Design review of the part built by this model. Coordinates are the model's own, in mm. Face numbers are marked on the shaded views. A direction names the side the tool comes from. Coordinates: 2 decimals unless noted, no trailing zeros. Order: outer loops, then holes, each group sorted by start corner. A loop starts at its lowest first (then second) coordinate and runs counter-clockwise, first axis right, second up. Notation, with made-up numbers: (9, 22.25) -> (35, 22.25) arc R31 ccw to (35, 48.25) -> close; hole circle Ø8 at (9, 8). An arc over 180 degrees is marked (long way). Write item = value, one per line.
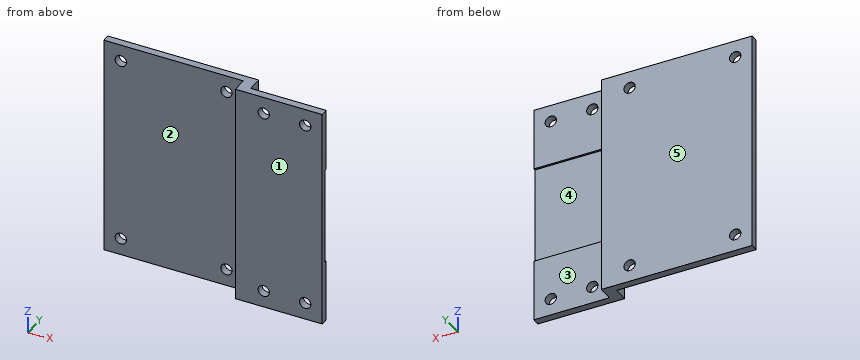
```python
from build123d import *

# Parameters (mm, degrees)
SKETCH_1_W          = 62
SKETCH_1_H          = 59
EXTRUDE_1_DEPTH     = 2
SKETCH_2_W          = 3
SKETCH_2_H          = 59
EXTRUDE_2_DEPTH     = 4
SKETCH_3_W          = 59
SKETCH_3_H          = 2
EXTRUDE_3_DEPTH     = 20
HOLE_WIZARD_M3_2_D  = 3
HOLE_WIZARD_M3_1_D  = 3
SKETCH_6_R          = 1.5
CUT_EXTRUDE_3_DEPTH = 10
SKETCH_7_W          = 59
SKETCH_7_H          = 2
CUT_EXTRUDE_4_DEPTH = 22
HOLE_WIZARD_M3_3_D  = 3
CUT_EXTRUDE_6_DEPTH = 0.5


with BuildPart() as part:
    # Sketch 1 → Extrude 1 (new body)
    with BuildSketch(Plane(origin=(0, 0, 0), x_dir=(1, 0, 0), z_dir=(0, 1, 0))):
        Rectangle(SKETCH_1_W, SKETCH_1_H)
    extrude(amount=EXTRUDE_1_DEPTH)

    # Sketch 2 → Extrude 2 (add)
    with BuildSketch(Plane.XZ):
        with Locations((29.5, 0)):
            Rectangle(SKETCH_2_W, SKETCH_2_H)
    extrude(amount=EXTRUDE_2_DEPTH)

    # Sketch 3 → Extrude 3 (add)
    with BuildSketch(Plane(origin=(31, 0, 0), x_dir=(0, 0, -1), z_dir=(1, 0, 0))):
        with Locations((0, -3)):
            Rectangle(SKETCH_3_W, SKETCH_3_H)
    extrude(amount=EXTRUDE_3_DEPTH)

    # Hole Wizard M3 _2 (through all)
    with Locations(Plane(origin=(23.5, 2, -25), x_dir=(0, 0, 1), z_dir=(0, 1, 0))):
        with Locations((0, 0), (50, 0)):
            Hole(HOLE_WIZARD_M3_2_D / 2)

    # Hole Wizard M3 _1 (through all)
    with Locations(Plane(origin=(35.5, -2, -25), x_dir=(0, 0, 1), z_dir=(0, 1, 0))):
        with Locations((0, 0), (0, 11), (50, 0), (50, 11)):
            Hole(HOLE_WIZARD_M3_1_D / 2)

    # Sketch 6 → Cut-Extrude 3 (cut)
    with BuildSketch(Plane(origin=(0, 2, 0), x_dir=(1, 0, 0), z_dir=(0, 1, 0))):
        with Locations(Location((-26.5, 25, 0), (0, 0, 270))):
            Circle(SKETCH_6_R)
        with Locations(Location((-26.5, -25, 0), (0, 0, 270))):
            Circle(SKETCH_6_R)
    extrude(amount=-CUT_EXTRUDE_3_DEPTH, mode=Mode.SUBTRACT)

    # Sketch 7 → Cut-Extrude 4 (cut)
    with BuildSketch(Plane.ZY.offset(31)):
        with Locations((0, 1)):
            Rectangle(SKETCH_7_W, SKETCH_7_H)
    extrude(amount=-CUT_EXTRUDE_4_DEPTH, mode=Mode.SUBTRACT)

    # Hole Wizard M3 _3 (through all)
    with Locations(Plane(origin=(-4.5, 2, -25), x_dir=(0, 0, 1), z_dir=(0, 1, 0))):
        with Locations((0, 0), (50, 0)):
            Hole(HOLE_WIZARD_M3_3_D / 2)

    # Sketch 9 → Cut-Extrude 6 (cut)
    with BuildSketch(Plane(origin=(0, -2, 0), x_dir=(1, 0, 0), z_dir=(0, 1, 0))):
        Polygon((51, -13), (51, 0), (51, 13), (31, 13), (31, -13), align=None)
    extrude(amount=-CUT_EXTRUDE_6_DEPTH, mode=Mode.SUBTRACT)


solid = part.part
```
(1) We need section D-D (z = 0.5). Write out the cut boundary in (x, y).
Report:
outline = (-9, 0) -> (28, 0) -> (28, -4) -> (51, -4) -> (51, -2.5) -> (31, -2.5) -> (31, 2) -> (-9, 2) -> close
(2) The part is to be moulded in two halves that separate along Z. For the marked faces 4 and 5, say which applies: released by +Z, released by -Z, zero draft, split by the parting line, or undercut.
Report:
face_4 = undercut
face_5 = zero draft
(3) We need section A-A (x = 35.5). Write out the cut boundary in (y, z), and give its area (3 significant figures).
Report:
outline = (-4, -29.5) -> (-2, -29.5) -> (-2, -26.5) -> (-4, -26.5) -> close; (-4, -23.5) -> (-2, -23.5) -> (-2, -13) -> (-2.5, -13) -> (-2.5, 13) -> (-2, 13) -> (-2, 23.5) -> (-4, 23.5) -> close; (-4, 26.5) -> (-2, 26.5) -> (-2, 29.5) -> (-4, 29.5) -> close
area = 93.0 mm²
(4) Insertion check: pin 1 (1.3 mm diameter, centred on y = 0.5, z = 6.5, fed in from +X); pin 2 (13 mm diameter, centred on x = 40, z = -23.5, fed in from +Y); pin 3 (2 mm diameter, centred on y = -1.5, z = 4.5, fed in from -X); pin 4 (2.5 mm diameter, centred on x = 23.5, z = 25, fed in from +Y). Each pin has a flat end and moves straight along its axis. Give the tip position at first contact, or say it passes through.
Report:
pin_1 = 31
pin_2 = -2
pin_3 = 28
pin_4 = through
(5) We need section C-C (y = 1.15). Write out the cut boundary in (x, z).
Report:
outline = (-9, -29.5) -> (31, -29.5) -> (31, 29.5) -> (-9, 29.5) -> close; hole circle Ø3 at (-4.5, -25); hole circle Ø3 at (-4.5, 25); hole circle Ø3 at (23.5, -25); hole circle Ø3 at (23.5, 25)
(6) We need section B-B (z = 25). Write out the cut boundary in (x, y), and give its area (3 significant figures).
Report:
outline = (-9, 0) -> (-6, 0) -> (-6, 2) -> (-9, 2) -> close; (-3, 0) -> (22, 0) -> (22, 2) -> (-3, 2) -> close; (25, 0) -> (28, 0) -> (28, -4) -> (34, -4) -> (34, -2) -> (31, -2) -> (31, 2) -> (25, 2) -> close; (37, -4) -> (45, -4) -> (45, -2) -> (37, -2) -> close; (48, -4) -> (51, -4) -> (51, -2) -> (48, -2) -> close
area = 108 mm²
(7) For L1, parallel to X at y = 1.5, z = 25; L2, parallel to X at y = -3.05, z = -25; L3, parallel to Y at x = 23, z = 0.5, list the stretches that pass through material, from the lowest coordinate up.
Report:
L1 = -9 to -6, -3 to 22, 25 to 31
L2 = 28 to 34, 37 to 45, 48 to 51
L3 = 0 to 2
(8) For the marked faces 1, 2 and 3, list the 3-axis set-ups (+Z, -Z, +X, -X, +Y, -Y) from which the entire face can be reached by the end or side of a thin tool; tool diameter is ignored.
Report:
face_1 = +Z, -Z, +X, -X, -Y
face_2 = +Z, -Z, -X, -Y
face_3 = +Z, -Z, +X, +Y
